from build123d import *

# Parameters (mm, degrees)
F1_DEPTH = 6.35
F3_DEPTH = 1.27
F5_DEPTH = 6.35
F6_R     = 12.827
F6_R_2   = 11.1125
F7_DEPTH = 6.35


with BuildPart() as f1:
    # F0 (on Top) → F1 (new body)
    with BuildSketch(Plane.XY):
        Polygon((50.8, 0), (12.7, 21.9970452561), (12.7, 0), (12.7, -21.9970452561), align=None)
        with BuildLine():
            ThreePointArc((36.5125, 0), (25.4, -11.1125), (14.2875, 0))
            ThreePointArc((14.2875, 0), (25.4, 11.1125), (36.5125, 0))
        make_face(mode=Mode.SUBTRACT)
        with BuildLine():
            Line((12.7, 0), (12.7, 21.9970452561))
            Line((12.7, 21.9970452561), (-6.35, 10.9985226281))
            Line((-6.35, 10.9985226281), (-5.55625, 9.6237072996))
            ThreePointArc((-5.55625, 9.6237072996), (5.55625, 9.6237072996), (11.1125, 0))
            Line((11.1125, 0), (12.7, 0))
        make_face()
        Polygon((-6.35, 10.9985226281), (12.7, 21.9970452561), (-25.4, 43.9940905122), (-25.4, 0), align=None)
        with BuildLine():
            ThreePointArc((-1.5875, 21.9970452561), (-3.0762927004, 16.4407952561), (-7.14375, 12.3733379566))
            ThreePointArc((-7.14375, 12.3733379566), (-22.3237072996, 27.5532952561), (-1.5875, 21.9970452561))
        make_face(mode=Mode.SUBTRACT)
        with BuildLine():
            Line((12.7, -21.9970452561), (12.7, 0))
            Line((12.7, 0), (11.1125, 0))
            ThreePointArc((11.1125, 0), (5.55625, -9.6237072996), (-5.55625, -9.6237072996))
            Line((-5.55625, -9.6237072996), (-6.35, -10.9985226281))
            Line((-6.35, -10.9985226281), (12.7, -21.9970452561))
        make_face()
        with BuildLine():
            Line((-5.55625, 9.6237072996), (-6.35, 10.9985226281))
            Line((-6.35, 10.9985226281), (-25.4, 0))
            Line((-25.4, 0), (-6.35, -10.9985226281))
            Line((-6.35, -10.9985226281), (-5.55625, -9.6237072996))
            ThreePointArc((-5.55625, -9.6237072996), (-11.1125, 0), (-5.55625, 9.6237072996))
        make_face()
        Polygon((-25.4, -43.9940905122), (12.7, -21.9970452561), (-6.35, -10.9985226281), (-25.4, 0), align=None)
        with BuildLine():
            ThreePointArc((-1.5875, -21.9970452561), (-22.3237072996, -27.5532952561), (-7.14375, -12.3733379566))
            ThreePointArc((-7.14375, -12.3733379566), (-3.0762927004, -16.4407952561), (-1.5875, -21.9970452561))
        make_face(mode=Mode.SUBTRACT)
    extrude(amount=F1_DEPTH)

    # F2 (on face) → F3 (cut)
    with BuildSketch(Plane.XY.offset(6.35)):
        Polygon((12.573, -21.7770748036), (12.573, 21.7770748036), (-25.146, 0), align=None)
        Polygon((-22.8768289089, 0), (11.4384144545, 19.8119149932), (11.4384144545, -19.8119149932), align=None, mode=Mode.SUBTRACT)
    extrude(amount=-F3_DEPTH, mode=Mode.SUBTRACT)

    # F4 (on face) → F5 (cut)
    with BuildSketch(Plane(origin=(0, 0, 0), x_dir=(1, 0, 0), z_dir=(0, 0, -1))):
        with BuildLine():
            Line((12.573, 2.54), (12.573, 21.7770748036))
            Line((12.573, 21.7770748036), (-4.0867954744, 12.1585374018))
            ThreePointArc((-4.0867954744, 12.1585374018), (6.4135, 11.1085078543), (12.573, 2.54))
        make_face()
        with BuildLine():
            ThreePointArc((12.827, 0), (12.7633420388, 1.2763342039), (12.573, 2.54))
            Line((12.573, 2.54), (12.573, -2.54))
            ThreePointArc((12.573, -2.54), (12.7633420388, -1.2763342039), (12.827, 0))
        make_face()
        with BuildLine():
            Line((12.573, -2.54), (12.573, 2.54))
            ThreePointArc((12.573, 2.54), (6.4135, 11.1085078543), (-4.0867954744, 12.1585374018))
            Line((-4.0867954744, 12.1585374018), (-8.4862045256, 9.6185374018))
            ThreePointArc((-8.4862045256, 9.6185374018), (-12.827, 0), (-8.4862045256, -9.6185374018))
            Line((-8.4862045256, -9.6185374018), (-4.0867954744, -12.1585374018))
            ThreePointArc((-4.0867954744, -12.1585374018), (6.4135, -11.1085078543), (12.573, -2.54))
        make_face()
        with BuildLine():
            Line((-8.4862045256, 9.6185374018), (-4.0867954744, 12.1585374018))
            ThreePointArc((-4.0867954744, 12.1585374018), (-6.4135, 11.1085078543), (-8.4862045256, 9.6185374018))
        make_face()
        with BuildLine():
            Line((12.573, -21.7770748036), (12.573, -2.54))
            ThreePointArc((12.573, -2.54), (6.4135, -11.1085078543), (-4.0867954744, -12.1585374018))
            Line((-4.0867954744, -12.1585374018), (12.573, -21.7770748036))
        make_face()
        with BuildLine():
            ThreePointArc((-8.4862045256, -9.6185374018), (-12.827, 0), (-8.4862045256, 9.6185374018))
            Line((-8.4862045256, 9.6185374018), (-25.146, 0))
            Line((-25.146, 0), (-8.4862045256, -9.6185374018))
        make_face()
        with BuildLine():
            ThreePointArc((-8.4862045256, -9.6185374018), (-6.4135, -11.1085078543), (-4.0867954744, -12.1585374018))
            Line((-4.0867954744, -12.1585374018), (-8.4862045256, -9.6185374018))
        make_face()
    extrude(amount=-F5_DEPTH, mode=Mode.SUBTRACT)

    # F6 (on face) → F7 (join)
    with BuildSketch(Plane(origin=(0, 0, 0), x_dir=(1, 0, 0), z_dir=(0, 0, -1))):
        Circle(F6_R)
        Circle(F6_R_2, mode=Mode.SUBTRACT)
    extrude(amount=-F7_DEPTH)


solid = f1.part
For this review, take the finished solid that the model builds, in its own axes (mm). Round coordinates to 2 decimals unless told otherwise and drop trailing zeros. Loops run counter-clockwise (first coordinate to the right, second up) from the corner with the lowest first, then second, coordinate; pieces in that order, holes last. Notation, with made-up numbers: (-31.5, -32) - (-19.5, -32) arc R26 ccw to (-19.5, -11) - close; hole circle Ø6 at (-19.5, 66.25). An arc over 180 degrees is marked (long way). One line per item, written item: value. Start each with the question number.
Item 1: Take a section at D-D (y = 1.5). Give the boundary of the cut face in (x, z).
Item 2: Clearance check with flat-ended pins moving along their axes: pin 1 Ø3 at (y, z) = (-20.5, 1) entering from +X; pin 2 Ø10 at (x, y) = (-14.5, 5) entering from -Z; pin 3 Ø2 at (y, z) = (-21, 2.5) entering from +X. State where each tip first meets the part, or that it passes through.
Item 3: Take a section at C-C (x = -18). Give the boundary of the cut face in (y, z), plus the area to 3 significant figures.
Item 4: Take a section at B-B (y = -23.5). Give the boundary of the cut face in (x, z).
Item 5: For L1, parallel to Y at x = -17, z = 1; L2, parallel to X at y = -0.5, z = 5.5; L3, parallel to Y at x = 0, z = 4, list the stretches that pass through material, from the lowest coordinate up.
Item 6: The part is to be moulded in two halves that separate along X. For faces 1 (the cylindrical face through (14.8, 3.34, 3.13)), 2 (the flat face through (12.167, -22.305, 3.131)), 3 (the flat face through (-10, -7, 0)), 4 (the flat face through (-25.4, 1, 3)), say which applies: +X half, -X half, draft (parallel to the pull), parting line (faces both ways), or undercut.
Item 7: Take a section at A-A (z = 1.5). Give the boundary of the cut face in (x, y) (1 decimal).
Answer below:
1. outline: (-25.4, 0) - (-22.55, 0) - (-22.55, 6.35) - (-25.4, 6.35) - close; (-12.74, 0) - (-11.01, 0) - (-11.01, 6.35) - (-12.74, 6.35) - close; (11.01, 0) - (14.39, 0) - (14.39, 6.35) - (11.01, 6.35) - close; (36.41, 0) - (48.2, 0) - (48.2, 6.35) - (36.41, 6.35) - close
2. pin 1: stops at x = 17.89
2. pin 2: stops at z = 0
2. pin 3: stops at x = 16.16
3. outline: (-39.72, 0) - (-31.76, 0) - (-31.76, 6.35) - (-39.72, 6.35) - close; (-12.23, 0) - (-4.13, 0) - (-4.13, 6.35) - (-12.23, 6.35) - close; (4.13, 0) - (12.23, 0) - (12.23, 6.35) - (4.13, 6.35) - close; (31.76, 0) - (39.72, 0) - (39.72, 6.35) - (31.76, 6.35) - close
3. area: 204 mm2
4. outline: (-25.4, 0) - (-23.71, 0) - (-23.71, 6.35) - (-25.4, 6.35) - close; (-1.69, 0) - (10.1, 0) - (10.1, 6.35) - (-1.69, 6.35) - close
5. L1: y = -39.14 to -32.24, -11.75 to -4.7, 4.7 to 11.75, 32.24 to 39.14
5. L2: x = -25.4 to -24.28, -12.82 to -11.1, 11.1 to 14.3, 36.5 to 49.93
5. L3: y = -29.33 to -14.52, -12.83 to -11.11, 11.11 to 12.83, 14.52 to 29.33
6. face 1: undercut
6. face 2: +X half
6. face 3: draft
6. face 4: -X half
7. outline: (-25.4, -44) - (50.8, 0) - (-25.4, 44) - close; hole (-25.1, 0) - (-8.5, -9.6) arc R12.8 cw to (-8.5, 9.6) - close; hole circle Ø22.2 at (-12.7, -22); hole circle Ø22.2 at (-12.7, 22); hole circle Ø22.2 at (0, 0); hole (-4.1, -12.2) - (12.6, -21.8) - (12.6, -2.5) arc R12.8 cw to start; hole (-4.1, 12.2) arc R12.8 cw to (12.6, 2.5) - (12.6, 21.8) - close; hole circle Ø22.2 at (25.4, 0)
